Read the model definition and answer for the solid it produces. Units are mm, in the model's axes. Round coordinates to 2 decimals unless told otherwise and drop trailing zeros. Order: outer loops, then holes, each group sorted by start corner. A loop starts at its lowest first (then second) coordinate and runs counter-clockwise, first axis right, second up. Notation, with made-up numbers: (58, 71.5) -> (72, 71.5) arc R19 cw to (72, 94.5) -> close; hole circle Ø3 at (88.25, -14.75). An arc over 180 degrees is marked (long way). Answer as a JSON object with one key per item and string values. Group by question number.
Item 1: Section B-B, the plane y = 2.25 is taken. Write down the section's boundary in (x, z).
Item 2: Given P1, Ø3.5, axis at y = 6.5, z = 10, coming from the -X side; P2, Ø0.5, axis at x = 2, z = 9, coming from the +Y side, each flat-ended and moving along its own axis, determine where each tip first touches the part or whether it passes through.
Item 3: Section C-C, the plane y = 6.5 is taken. Write down the section's boundary in (x, z), plus the area to 3 significant figures.
Item 4: Section A-A, the plane z = 10 is taken. Write down the section's boundary in (x, y).
Item 5: Consider probe 1 along Y at (x, z) = (3.35, 10); probe 2 along X at (y, z) = (12.25, 13.5); probe 3 along Z at (x, y) = (3.7, 5). Determine where each line is inside the solid, lowest interval first. Write a range as from..to.
Item 6: Section D-D, the plane z = 7.25 is taken. Write down the section's boundary in (x, y), plus the area to 3 significant figures.
from build123d import *

# Parameters (mm, degrees)
BOSS_EXTRUDE1_DEPTH = 20
CUT_EXTRUDE1_REACH  = 26.312
SKETCH2_R           = 1.85


with BuildPart() as part:
    # Sketch1 → Boss-Extrude1 (new body)
    with BuildSketch(Plane.XY):
        with BuildLine():
            Line((3.22, 13.22), (3.64, 13.22))
            ThreePointArc((3.64, 13.22), (3.922842712, 13.102842712), (4.04, 12.82))
            Line((4.04, 12.82), (4.04, 0.4))
            ThreePointArc((4.04, 0.4), (3.922842712, 0.117157288), (3.64, 0))
            Line((3.64, 0), (0.4, 0))
            ThreePointArc((0.4, 0), (0.117157288, 0.117157288), (0, 0.4))
            Line((0, 0.4), (0, 12.82))
            ThreePointArc((0, 12.82), (0.117157288, 13.102842712), (0.4, 13.22))
            Line((0.4, 13.22), (0.82, 13.22))
            ThreePointArc((0.82, 13.22), (1.102842712, 13.102842712), (1.22, 12.82))
            Line((1.22, 12.82), (1.22, 1.22))
            Line((1.22, 1.22), (2.82, 1.22))
            Line((2.82, 1.22), (2.82, 12.82))
            ThreePointArc((2.82, 12.82), (2.937157288, 13.102842712), (3.22, 13.22))
        make_face()
    extrude(amount=BOSS_EXTRUDE1_DEPTH)

    # Cut-Extrude1: up to this face of the body (flat: up to its plane)
    cut_extrude1_end = Plane(part.part.faces().sort_by_distance((4.04, 6.61, 10))[0])
    # Sketch2 → Cut-Extrude1 (cut, up to the picked face)
    with BuildSketch(Plane.ZY, mode=Mode.PRIVATE) as cut_extrude1_sk1:
        with Locations((10, 6.5)):
            Circle(SKETCH2_R)
    cut_extrude1_tool1 = split(extrude(cut_extrude1_sk1.sketch, amount=-CUT_EXTRUDE1_REACH, mode=Mode.PRIVATE), bisect_by=cut_extrude1_end, keep=Keep.BOTH, mode=Mode.PRIVATE)
    add(cut_extrude1_tool1.solids().sort_by(Axis((0, 6.5, 10), (1, 0, 0)))[0], mode=Mode.SUBTRACT)


solid = part.part
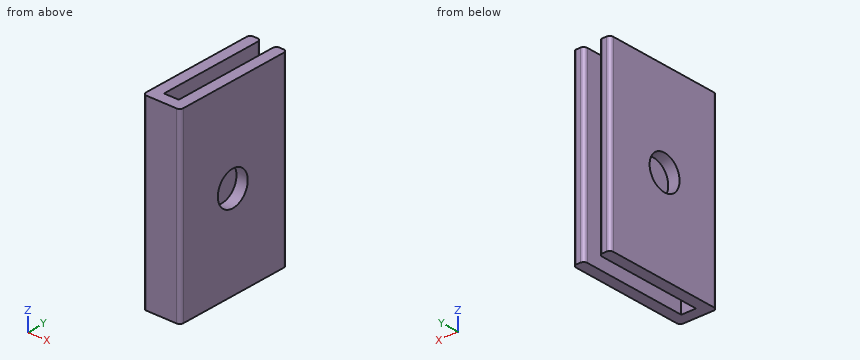
Values found:
{
 "1": {"outline": "(0, 0) -> (1.22, 0) -> (1.22, 20) -> (0, 20) -> close; (2.82, 0) -> (4.04, 0) -> (4.04, 20) -> (2.82, 20) -> close"},
 "2": {"P1": "through", "P2": "y = 1.22"},
 "3": {"outline": "(0, 0) -> (1.22, 0) -> (1.22, 8.15) -> (0, 8.15) -> close; (0, 11.85) -> (1.22, 11.85) -> (1.22, 20) -> (0, 20) -> close; (2.82, 0) -> (4.04, 0) -> (4.04, 8.15) -> (2.82, 8.15) -> close; (2.82, 11.85) -> (4.04, 11.85) -> (4.04, 20) -> (2.82, 20) -> close", "area": "39.8 mm2"},
 "4": {"outline": "(0, 0.4) arc R0.4 ccw to (0.4, 0) -> (3.64, 0) arc R0.4 ccw to (4.04, 0.4) -> (4.04, 4.65) -> (2.82, 4.65) -> (2.82, 1.22) -> (1.22, 1.22) -> (1.22, 4.65) -> (0, 4.65) -> close; (0, 8.35) -> (1.22, 8.35) -> (1.22, 12.82) arc R0.4 ccw to (0.82, 13.22) -> (0.4, 13.22) arc R0.4 ccw to (0, 12.82) -> close; (2.82, 8.35) -> (4.04, 8.35) -> (4.04, 12.82) arc R0.4 ccw to (3.64, 13.22) -> (3.22, 13.22) arc R0.4 ccw to (2.82, 12.82) -> close"},
 "5": {"probe 1": "0..4.65, 8.35..13.22", "probe 2": "0..1.22, 2.82..4.04", "probe 3": "0..8.92, 11.08..20"},
 "6": {"outline": "(0, 0.4) arc R0.4 ccw to (0.4, 0) -> (3.64, 0) arc R0.4 ccw to (4.04, 0.4) -> (4.04, 12.82) arc R0.4 ccw to (3.64, 13.22) -> (3.22, 13.22) arc R0.4 ccw to (2.82, 12.82) -> (2.82, 1.22) -> (1.22, 1.22) -> (1.22, 12.82) arc R0.4 ccw to (0.82, 13.22) -> (0.4, 13.22) arc R0.4 ccw to (0, 12.82) -> close", "area": "34.0 mm2"}
}
